Could you check a few things on this model? Use its own coordinates, in mm. Give positions to 0.01 mm unless a question says otherwise; leave off trailing zeros. Loops run counter-clockwise (first coordinate to the right, second up) from the corner with the lowest first, then second, coordinate; pieces in that order, holes last. Notation, with made-up numbers: M 23,-10 L 34,-10 A10 ccw 34,1 Z; hole C 52.5,38 d3. An arc over 180 degrees is marked long. Return JSON: item names as keys, results as strings. Group by question number.
1. If we section it at D-D (z = 10): Write out the boundary of the cut face in (x, y), plus the area to 3 significant figures.
2. Please list where these lines run through material, in increasing order: line 1 (X direction, y = 1.5, z = 7); line 2 (Y direction, x = -12.7, z = 9); line 3 (X direction, y = -4.5, z = 7.75).
3. If we section it at A-A (z = 7): Write out the boundary of the cut face in (x, y), plus the area to 3 significant figures.
4. If we section it at C-C (y = 0): Write out the boundary of the cut face in (x, z), plus the area to 3 significant figures.
5. If we mould it in two halves opening along Y, with no side actions, what happens to faces 1 (the cylindrical face through (-11.56, 0.05, 7.4)), 2 (the flat face through (0, -6, 7)), 3 (the flat face through (0, -2, 15))? For each: +Y half, -Y half, draft (parallel to the pull), parting line (faces both ways), or undercut.
6. If we section it at B-B (x = -12.7): Write out the boundary of the cut face in (y, z), plus the area to 3 significant figures.
```python
from build123d import *

# Parameters (mm, degrees)
SKETCH1_W           = 53
SKETCH1_H           = 12
BOSS_EXTRUDE1_DEPTH = 15
CUT_EXTRUDE1_REACH  = 34.73
SKETCH2_R           = 1.143
FILLET1_R           = 2
SKETCH3_R           = 1.143
CUT_EXTRUDE2_DEPTH  = 32.036269106


with BuildPart() as part:
    # Sketch1 → Boss-Extrude1 (new body)
    with BuildSketch(Plane.XY):
        Rectangle(SKETCH1_W, SKETCH1_H)
    extrude(amount=BOSS_EXTRUDE1_DEPTH)

    # Sketch2 → Cut-Extrude1 (cut, up to next)
    with BuildSketch(Plane.XZ.offset(6), mode=Mode.PRIVATE) as cut_extrude1_sk1:
        with Locations(Location((-19.05, 7, 0), (0, 0, 270))):
            Circle(SKETCH2_R)
    cut_extrude1_tool1 = extrude(cut_extrude1_sk1.sketch, amount=-CUT_EXTRUDE1_REACH, mode=Mode.PRIVATE) & part.part
    # Sketch2 → Cut-Extrude1 (cut, up to next)
    with BuildSketch(Plane.XZ.offset(6), mode=Mode.PRIVATE) as cut_extrude1_sk2:
        with Locations(Location((19.05, 7, 0), (0, 0, 270))):
            Circle(SKETCH2_R)
    cut_extrude1_tool2 = extrude(cut_extrude1_sk2.sketch, amount=-CUT_EXTRUDE1_REACH, mode=Mode.PRIVATE) & part.part
    add(cut_extrude1_tool1.solids().sort_by_distance((-19.05, -6, 7))[0], mode=Mode.SUBTRACT)
    add(cut_extrude1_tool2.solids().sort_by_distance((19.05, -6, 7))[0], mode=Mode.SUBTRACT)

    # Fillet1
    fillet1_edges = [part.edges().sort_by_distance(p)[0] for p in [
        (-26.5, 0, 15),
        (26.5, 0, 15),
        (0, 6, 15),
        (26.5, -6, 7.5),
        (-26.5, -6, 7.5),
        (-26.5, 6, 7.5),
        (26.5, 6, 7.5),
    ]]
    fillet(fillet1_edges, radius=FILLET1_R)

    # Sketch3 → Cut-Extrude2 (cut, through all)
    with BuildSketch(Plane(origin=(0, 0, 0), x_dir=(-1, 0, 0), z_dir=(0, 0, -1))):
        with Locations((-12.7, 0)):
            Circle(SKETCH3_R)
        with Locations((12.7, 0)):
            Circle(SKETCH3_R)
        Circle(SKETCH3_R)
    extrude(amount=-CUT_EXTRUDE2_DEPTH, mode=Mode.SUBTRACT)


solid = part.part
```
Answer:
{
 "1": {"outline": "M -26.5,-4 A2 ccw -24.5,-6 L 24.5,-6 A2 ccw 26.5,-4 L 26.5,4 A2 ccw 24.5,6 L -24.5,6 A2 ccw -26.5,4 Z; hole C -12.7,0 d2.29; hole C 0,0 d2.29; hole C 12.7,0 d2.29", "area": "620 mm²"},
 "2": {"line 1": "x = -26.5 to -20.19, -17.91 to 17.91, 20.19 to 26.5", "line 2": "y = -6 to -1.14, 1.14 to 6", "line 3": "x = -26.44 to -19.91, -18.19 to 18.19, 19.91 to 26.44"},
 "3": {"outline": "M -26.5,-4 A2 ccw -24.5,-6 L -20.19,-6 L -20.19,6 L -24.5,6 A2 ccw -26.5,4 Z; M -17.91,-6 L 17.91,-6 L 17.91,6 L -17.91,6 Z; M 20.19,-6 L 24.5,-6 A2 ccw 26.5,-4 L 26.5,4 A2 ccw 24.5,6 L 20.19,6 Z; hole C -12.7,0 d2.29; hole C 0,0 d2.29; hole C 12.7,0 d2.29", "area": "565 mm²"},
 "4": {"outline": "M -26.5,0 L -13.84,0 L -13.84,15 L -24.5,15 A2 ccw -26.5,13 Z; M -11.56,0 L -1.14,0 L -1.14,15 L -11.56,15 Z; M 1.14,0 L 11.56,0 L 11.56,15 L 1.14,15 Z; M 13.84,0 L 26.5,0 L 26.5,13 A2 ccw 24.5,15 L 13.84,15 Z; hole C -19.05,7 d2.29; hole C 19.05,7 d2.29", "area": "682 mm²"},
 "5": {"face 1": "undercut", "face 2": "-Y half", "face 3": "draft"},
 "6": {"outline": "M -6,0 L -1.14,0 L -1.14,15 L -6,15 Z; M 1.14,0 L 6,0 L 6,13 A2 ccw 4,15 L 1.14,15 Z", "area": "145 mm²"}
}
